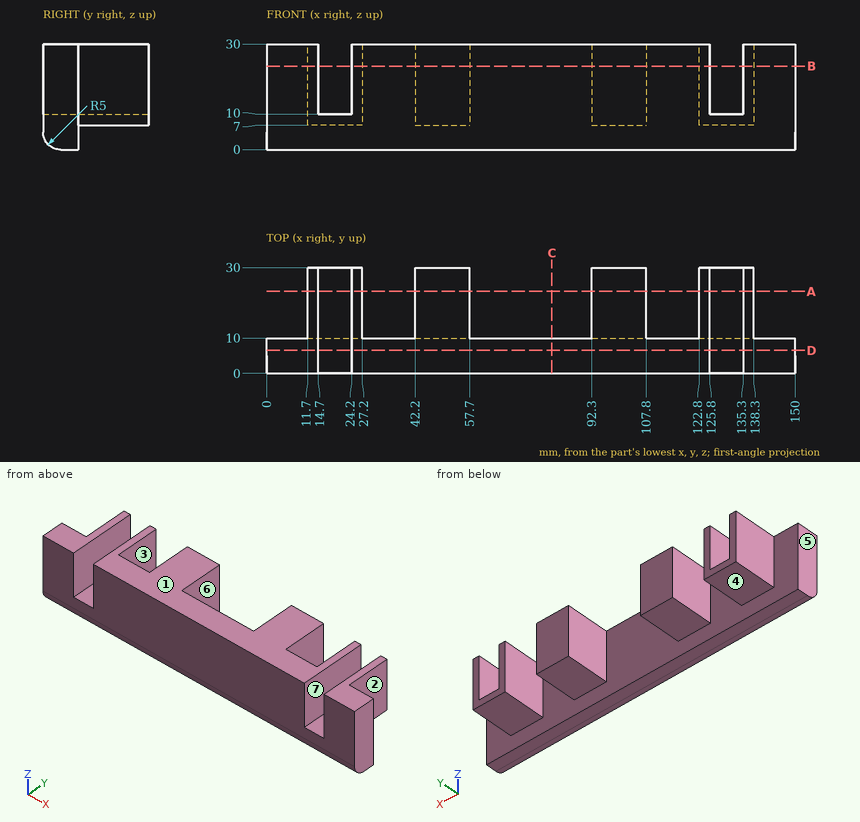
For this review, use the dimensioned drawing (mm, ordinates from the lowest corner) and the shaded views. A direction names the side the tool comes from. Give positions to 0.01 mm unless a question says otherwise; leave off trailing zeros. Write each loop counter-clockwise with the first axis right and the second up, starting at its lowest first coordinate (ties: lowest second). Pieces come first, ordered by that corner, then holes.
(1) Consider section D-D, the plane y = 6.5. Give the boundary of the cut face in (x, z), and give its area (3 significant figures).
(2) Consider section A-A, the plane y = 23.25. Give the boundary of the cut face in (x, z).
(3) Consider section B-B, the plane z = 23.75. Give the boundary of the cut face in (x, y), and give its area (3 significant figures).
(4) The part is to be moulded in two halves that separate along X. For the marked faces 1, 2 and 3, say which applies: released by +X, released by -X, zero draft, split by the parting line, or undercut.
(5) Consider section C-C, the plane x = 81. Give the boundary of the cut face in (y, z).
(6) For P1, Ø3, axis at y = 23.5, z = 4.5, coming from the -X side; P2, Ø10, axis at y = 17.5, z = 15.5, coming from the +X side; P3, Ø8, axis at x = 132.5, y = 23.5, coming from the -Z side; P4, Ø6, axis at y = 24, z = 17.5, coming from the -X side, all flat-tipped, find the tip position at first contact; note any pin that passes through.
(7) Tool access review of the marked faces 4, 5, 6 and 7: name each direction out of +Z, -Z, +X, -X, +Y, -Y from which nothing blocks a thin tool from reaching the whole face with its end or side.
(8) To check wall thickness, follow L1, parallel to X at y = 10.25, z = 24.5; L2, parallel to X at y = 25.5, z = 7.75; L3, parallel to Y at x = 89.5, z = 24.5. State the ranges of each line that lie inside material, in increasing order.
Returned:
1. outline: (0, 0) - (150, 0) - (150, 30) - (135.3, 30) - (135.3, 10) - (125.8, 10) - (125.8, 30) - (24.2, 30) - (24.2, 10) - (14.7, 10) - (14.7, 30) - (0, 30) - close
1. area: 4,120 mm2
2. outline: (11.7, 7) - (27.2, 7) - (27.2, 30) - (24.2, 30) - (24.2, 10) - (14.7, 10) - (14.7, 30) - (11.7, 30) - close; (42.2, 7) - (57.7, 7) - (57.7, 30) - (42.2, 30) - close; (92.3, 7) - (107.8, 7) - (107.8, 30) - (92.3, 30) - close; (122.8, 7) - (138.3, 7) - (138.3, 30) - (135.3, 30) - (135.3, 10) - (125.8, 10) - (125.8, 30) - (122.8, 30) - close
3. outline: (0, 0) - (14.7, 0) - (14.7, 30) - (11.7, 30) - (11.7, 10) - (0, 10) - close; (24.2, 0) - (125.8, 0) - (125.8, 30) - (122.8, 30) - (122.8, 10) - (107.8, 10) - (107.8, 30) - (92.3, 30) - (92.3, 10) - (57.7, 10) - (57.7, 30) - (42.2, 30) - (42.2, 10) - (27.2, 10) - (27.2, 30) - (24.2, 30) - close; (135.3, 0) - (150, 0) - (150, 10) - (138.3, 10) - (138.3, 30) - (135.3, 30) - close
3. area: 2,170 mm2
4. face 1: zero draft
4. face 2: released by +X
4. face 3: undercut
5. outline: (0, 5) arc R5 ccw to (5, 0) - (10, 0) - (10, 30) - (0, 30) - close
6. P1: passes through
6. P2: stops at x = 138.3
6. P3: stops at z = 7
6. P4: stops at x = 11.7
7. face 4: -Z, +X, -X, +Y
7. face 5: +Z, -Z, -X, +Y, -Y
7. face 6: +Z, -Z, +Y
7. face 7: +Z, +Y, -Y
8. L1: x = 11.7 to 14.7, 24.2 to 27.2, 42.2 to 57.7, 92.3 to 107.8, 122.8 to 125.8, 135.3 to 138.3
8. L2: x = 11.7 to 27.2, 42.2 to 57.7, 92.3 to 107.8, 122.8 to 138.3
8. L3: y = 0 to 10
